```python
from build123d import *

# Parameters (mm, degrees)
BOSS_EXTRUDE1_DEPTH = 3.175


with BuildPart() as part:
    # Sketch1 → Boss-Extrude1 (new body)
    with BuildSketch(Plane.XY):
        with BuildLine():
            Line((-266.475505146, 24.162932081), (-270.592467022, 23.5453878))
            ThreePointArc((-270.592467022, 23.5453878), (-274.462155482, 21.409374702), (-276.000505146, 17.265641959))
            Line((-276.000505146, 17.265641959), (-276.000505146, 7.017932081))
            ThreePointArc((-276.000505146, 7.017932081), (-274.140633206, 2.527804021), (-269.650505146, 0.667932081))
            Line((-269.650505146, 0.667932081), (-266.475505146, 0.667932081))
            Line((-266.475505146, 0.667932081), (-266.475505146, 10.034182081))
            ThreePointArc((-266.475505146, 10.034182081), (-268.856755146, 12.415432081), (-266.475505146, 14.796682081))
            Line((-266.475505146, 14.796682081), (-266.475505146, 24.162932081))
        make_face()
        with BuildLine():
            Line((-228.375505146, 29.877932081), (-266.475505146, 24.162932081))
            Line((-266.475505146, 24.162932081), (-266.475505146, 14.796682081))
            ThreePointArc((-266.475505146, 14.796682081), (-264.791707123, 14.099230104), (-264.094255146, 12.415432081))
            ThreePointArc((-264.094255146, 12.415432081), (-264.791707123, 10.731634059), (-266.475505146, 10.034182081))
            Line((-266.475505146, 10.034182081), (-266.475505146, 0.667932081))
            Line((-266.475505146, 0.667932081), (-250.600505146, 0.667932081))
            Line((-250.600505146, 0.667932081), (-250.600505146, 3.842932081))
            Line((-250.600505146, 3.842932081), (-237.900505146, 3.842932081))
            Line((-237.900505146, 3.842932081), (-237.900505146, 0.667932081))
            Line((-237.900505146, 0.667932081), (-228.375505146, 0.667932081))
            Line((-228.375505146, 0.667932081), (-228.375505146, 12.557716041))
            ThreePointArc((-228.375505146, 12.557716041), (-230.756755146, 14.938966041), (-228.375505146, 17.320216041))
            Line((-228.375505146, 17.320216041), (-228.375505146, 29.877932081))
        make_face()
        with BuildLine():
            Line((-226.142467022, 30.2128878), (-228.375505146, 29.877932081))
            Line((-228.375505146, 29.877932081), (-228.375505146, 17.320216041))
            ThreePointArc((-228.375505146, 17.320216041), (-226.691707123, 16.622764063), (-225.994255146, 14.938966041))
            ThreePointArc((-225.994255146, 14.938966041), (-226.691707123, 13.255168018), (-228.375505146, 12.557716041))
            Line((-228.375505146, 12.557716041), (-228.375505146, 0.667932081))
            Line((-228.375505146, 0.667932081), (-225.200505146, 0.667932081))
            ThreePointArc((-225.200505146, 0.667932081), (-220.710377085, 2.527804021), (-218.850505146, 7.017932081))
            Line((-218.850505146, 7.017932081), (-218.850505146, 23.933141959))
            ThreePointArc((-218.850505146, 23.933141959), (-221.056772403, 28.744792295), (-226.142467022, 30.2128878))
        make_face()
    extrude(amount=BOSS_EXTRUDE1_DEPTH)


solid = part.part
```
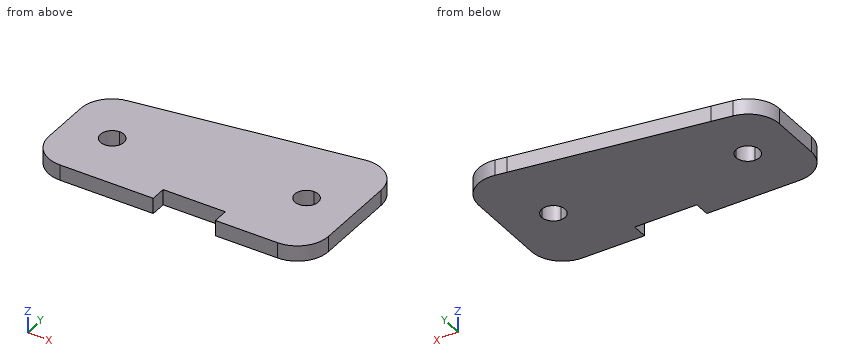
Read the model definition and answer for the solid it produces. Units are mm, in the model's axes. Coordinates: 2 decimals unless noted, no trailing zeros. Loops run counter-clockwise (first coordinate to the right, second up) from the corner with the lowest first, then second, coordinate; pieces in that order, holes last. Notation, with made-up numbers: (85.25, 70.5) -> (112.25, 70.5) arc R11 ccw to (112.25, 75.5) -> close; hole circle Ø5 at (71, 17). An arc over 180 degrees is marked (long way). Return JSON: item names as keys, results as strings.
Item 1: Find section C-C (y = 4.5). Determine the outline of the cut face in (x, z) (3 decimals).
Answers:
{"outline": "(-275.48, 0) -> (-219.371, 0) -> (-219.371, 3.175) -> (-275.48, 3.175) -> close"}
Item 2: Find section A-A (z = 1.55). Determine the outline of the cut face in (x, y).
Answers:
{"outline": "(-276, 7.02) arc R6.35 ccw to (-269.65, 0.67) -> (-250.6, 0.67) -> (-250.6, 3.84) -> (-237.9, 3.84) -> (-237.9, 0.67) -> (-225.2, 0.67) arc R6.35 ccw to (-218.85, 7.02) -> (-218.85, 23.93) arc R6.35 ccw to (-226.14, 30.21) -> (-270.59, 23.55) arc R6.35 ccw to (-276, 17.27) -> close; hole circle Ø4.76 at (-266.48, 12.42); hole circle Ø4.76 at (-228.38, 14.94)"}
Item 3: Find the intervals of material crossed by probe 1 along Y at (x, z) = (-245, 2.4); probe 2 along X at (y, z) = (18, 2.3); probe 3 along X at (y, z) = (10.5, 2.4), in increasing order.
Answers:
{"probe 1": "y = 3.84 to 27.38", "probe 2": "x = -275.96 to -218.85", "probe 3": "x = -276 to -267.89, -265.06 to -218.85"}
Item 4: Flat-ended cylindrical pins translate along their axes: P1, Ø1, axis at y = 2, z = 2, coming from the -X side; P2, Ø1, axis at y = 2.5, z = 1.5, coming from the +X side. Find the tip coordinate at first contact, or state that the pin passes through.
Answers:
{"P1": "stops at x = -274.11", "P2": "stops at x = -220.28"}
Item 5: Find section B-B (x = -267). Determine the outline of the cut face in (y, z) (3 decimals).
Answers:
{"outline": "(0.668, 0) -> (10.093, 0) -> (10.093, 3.175) -> (0.668, 3.175) -> close; (14.738, 0) -> (24.084, 0) -> (24.084, 3.175) -> (14.738, 3.175) -> close"}
Item 6: Find section D-D (x = -242.5). Determine the outline of the cut face in (y, z) (3 decimals), plus the area to 3 significant figures.
Answers:
{"outline": "(3.843, 0) -> (27.759, 0) -> (27.759, 3.175) -> (3.843, 3.175) -> close", "area": "75.9 mm2"}
